Read the model definition and answer for the solid it produces. Units are mm, in the model's axes. A direction names the side the tool comes from. Give positions to 0.01 mm unless a question says otherwise; leave off trailing zeros. Loops run counter-clockwise (first coordinate to the right, second up) from the corner with the lowest first, then second, coordinate; pieces in that order, holes last. Notation, with made-up numbers: M 78,71.25 L 94,71.25 A29 ccw 94,109.25 Z; hole C -30,-38.5 d1. An arc over 180 degrees is marked long. Return JSON: item names as keys, results as strings. Group by question number.
```python
from build123d import *
from build123d.topology import SkipClean

# Parameters (mm, degrees)
BOSS_EXTRUDE1_DEPTH     = 15.875
CUT_EXTRUDE2_START      = -11.875
CUT_EXTRUDE2_DEPTH      = 11.875
M4_CLEARANCE_HOLE1_D    = 4.5
CHAMFER1_SIZE           = 4.7625
SHELL1_OUTLINE_R        = 20.45
SHELL1_DEPTH            = 10.284072775
SHELL1_2_DEPTH          = 2
BOSS_EXTRUDE2_START     = 2
BOSS_EXTRUDE2_DEPTH     = 2
SKETCH7_W               = 7.14375
SKETCH7_H               = 4.7625
SKETCH7_W_2             = 4.7625
SKETCH7_H_2             = 7.14375
CUT_EXTRUDE5_DEPTH      = 0.5
CUT_EXTRUDE7_DEPTH      = 42.774640932
CUT_EXTRUDE7_DEPTH_BACK = 42.774640932
SKETCH9_W               = 6.175
SKETCH9_H               = 19.378
SKETCH9_W_2             = 3.175
SKETCH9_H_2             = 16.378
SKETCH9_W_3             = 1.5018
SKETCH12_R              = 1.27
CUT_EXTRUDE10_DEPTH     = 42.774640932


with BuildPart() as part:
    # Sketch1 → Boss-Extrude1 (new body)
    with BuildSketch(Plane.XY):
        with BuildLine():
            ThreePointArc((-9.919608253, 20.139609532), (-22.45, 0), (-9.919608253, -20.139609532))
            ThreePointArc((-9.919608253, -20.139609532), (-6.265793461, -23.208178662), (-4.449768206, -27.62049453))
            ThreePointArc((-4.449768206, -27.62049453), (0, -31.45), (4.449768206, -27.62049453))
            ThreePointArc((4.449768206, -27.62049453), (6.265793461, -23.208178662), (9.919608253, -20.139609532))
            ThreePointArc((9.919608253, -20.139609532), (22.45, 0), (9.919608253, 20.139609532))
            ThreePointArc((9.919608253, 20.139609532), (6.265793461, 23.208178662), (4.449768206, 27.62049453))
            ThreePointArc((4.449768206, 27.62049453), (0, 31.45), (-4.449768206, 27.62049453))
            ThreePointArc((-4.449768206, 27.62049453), (-6.265793461, 23.208178662), (-9.919608253, 20.139609532))
        make_face()
    extrude(amount=BOSS_EXTRUDE1_DEPTH)

    # Sketch3 → Cut-Extrude2 (cut)
    with SkipClean():  # the faces are left unmerged after this step: merging them gives an invalid solid
        with BuildSketch(Plane.XY.offset(15.875).offset(CUT_EXTRUDE2_START)):
            with BuildLine():
                ThreePointArc((-4.449768206, 27.62049453), (-6.265793461, 23.208178662), (-9.919608253, 20.139609532))
                ThreePointArc((-9.919608253, 20.139609532), (0, 22.45), (9.919608253, 20.139609532))
                ThreePointArc((9.919608253, 20.139609532), (6.265793461, 23.208178662), (4.449768206, 27.62049453))
                ThreePointArc((4.449768206, 27.62049453), (0, 31.45), (-4.449768206, 27.62049453))
            make_face()
            with BuildLine():
                ThreePointArc((9.919608253, -20.139609532), (0, -22.45), (-9.919608253, -20.139609532))
                ThreePointArc((-9.919608253, -20.139609532), (-6.265793461, -23.208178662), (-4.449768206, -27.62049453))
                ThreePointArc((-4.449768206, -27.62049453), (0, -31.45), (4.449768206, -27.62049453))
                ThreePointArc((4.449768206, -27.62049453), (6.265793461, -23.208178662), (9.919608253, -20.139609532))
            make_face()
        extrude(amount=CUT_EXTRUDE2_DEPTH, mode=Mode.SUBTRACT)

    # M4 Clearance Hole1 (through all)
    with Locations(Plane.XY.offset(4)):
        with Locations((0, -26.95), (0, 26.95)):
            Hole(M4_CLEARANCE_HOLE1_D / 2)

    # Chamfer1
    chamfer1_edges = [part.edges().sort_by_distance(p)[0] for p in [
        (22.45, 0, 15.875),
    ]]
    chamfer(chamfer1_edges, length=CHAMFER1_SIZE)

    # Shell1: read off the stored shape, not the designer's step
    # Shell1 outline → Shell1 (cut)
    with SkipClean():  # the faces are left unmerged after this step: merging them gives an invalid solid
        with BuildSketch(Plane.XY):
            Circle(SHELL1_OUTLINE_R)
        extrude(amount=SHELL1_DEPTH, mode=Mode.SUBTRACT)

    # Shell1 2 outline → Shell1 2 (cut)
    with SkipClean():  # the faces are left unmerged after this step: merging them gives an invalid solid
        with BuildSketch(Plane.XY):
            with BuildLine():
                ThreePointArc((-3.336769132, -24.317800965), (0, -22.7), (3.336769132, -24.317800965))
                ThreePointArc((3.336769132, -24.317800965), (5.656595992, -20.826114024), (9.035901505, -18.345434963))
                ThreePointArc((9.035901505, -18.345434963), (0, -20.45), (-9.035901505, -18.345434963))
                ThreePointArc((-9.035901505, -18.345434963), (-5.656595992, -20.826114024), (-3.336769132, -24.317800965))
            make_face()
            with BuildLine():
                ThreePointArc((-3.336769132, 24.317800965), (-5.656595992, 20.826114024), (-9.035901505, 18.345434963))
                ThreePointArc((-9.035901505, 18.345434963), (0, 20.45), (9.035901505, 18.345434963))
                ThreePointArc((9.035901505, 18.345434963), (5.656595992, 20.826114024), (3.336769132, 24.317800965))
                ThreePointArc((3.336769132, 24.317800965), (0, 22.7), (-3.336769132, 24.317800965))
            make_face()
        extrude(amount=SHELL1_2_DEPTH, mode=Mode.SUBTRACT)

    # Shell1 3 outline → Shell1 3 (revolve, cut)
    with SkipClean():  # the faces are left unmerged after this step: merging them gives an invalid solid
        with BuildSketch(Plane.XZ):
            Polygon((16.859072875, 13.875), (0, 13.875), (0, 10.284072775), (20.45, 10.284072775), align=None)
        revolve(axis=Axis((0, 0, 0), (0, 0, 1)), mode=Mode.SUBTRACT)

    # Sketch6 → Boss-Extrude2 (add)
    with SkipClean():  # the faces are left unmerged after this step: merging them gives an invalid solid
        with BuildSketch(Plane(origin=(0, 0, 2), x_dir=(-1, 0, 0), z_dir=(0, 0, -1)).offset(BOSS_EXTRUDE2_START)):
            with BuildLine():
                ThreePointArc((3.336769132, -24.317800965), (0, -22.7), (-3.336769132, -24.317800965))
                ThreePointArc((-3.336769132, -24.317800965), (-5.656595992, -20.826114024), (-9.035901505, -18.345434963))
                ThreePointArc((-9.035901505, -18.345434963), (0, -20.45), (9.035901505, -18.345434963))
                ThreePointArc((9.035901505, -18.345434963), (5.656595992, -20.826114024), (3.336769132, -24.317800965))
            make_face()
            with BuildLine():
                ThreePointArc((-9.035901505, 18.345434963), (-5.656595992, 20.826114024), (-3.336769132, 24.317800965))
                ThreePointArc((-3.336769132, 24.317800965), (0, 22.7), (3.336769132, 24.317800965))
                ThreePointArc((3.336769132, 24.317800965), (5.656595992, 20.826114024), (9.035901505, 18.345434963))
                ThreePointArc((9.035901505, 18.345434963), (0, 20.45), (-9.035901505, 18.345434963))
            make_face()
        extrude(amount=-BOSS_EXTRUDE2_DEPTH)

    # Sketch7 → Cut-Extrude5 (cut)
    with SkipClean():  # the faces are left unmerged after this step: merging them gives an invalid solid
        with BuildSketch(Plane.XY.offset(15.875)):
            with Locations((-5.953125, 0)):
                Rectangle(SKETCH7_W, SKETCH7_H)
            Rectangle(SKETCH7_W_2, SKETCH7_H)
            with Locations((5.953125, 0)):
                Rectangle(SKETCH7_W, SKETCH7_H)
            with Locations((0, -5.953125)):
                Rectangle(SKETCH7_W_2, SKETCH7_H_2)
            with Locations((0, 5.953125)):
                Rectangle(SKETCH7_W_2, SKETCH7_H_2)
        extrude(amount=-CUT_EXTRUDE5_DEPTH, mode=Mode.SUBTRACT)

    # Sketch9 → Cut-Extrude7 (cut, two sides: drawn at the far end of the back side and taken through both)
    # profile 1 of 3: a face of its own
    with SkipClean():  # the faces are left unmerged after this step: merging them gives an invalid solid
        with BuildSketch(Plane(origin=(0, 0, 0), x_dir=(0, 0, -1), z_dir=(1, 0, 0)).offset(-CUT_EXTRUDE7_DEPTH_BACK)):
            with Locations((-4.5893, 0)):
                Rectangle(SKETCH9_W, SKETCH9_H)
            with Locations((-4.5893, 0)):
                Rectangle(SKETCH9_W_2, SKETCH9_H_2, mode=Mode.SUBTRACT)
        # profile 2 of 3: a face of its own
        with BuildSketch(Plane(origin=(0, 0, 0), x_dir=(0, 0, -1), z_dir=(1, 0, 0)).offset(-CUT_EXTRUDE7_DEPTH_BACK)):
            with Locations((-0.7509, 0)):
                Rectangle(SKETCH9_W_3, SKETCH9_H)
        # profile 3 of 3: a face of its own
        with BuildSketch(Plane(origin=(0, 0, 0), x_dir=(0, 0, -1), z_dir=(1, 0, 0)).offset(-CUT_EXTRUDE7_DEPTH_BACK)):
            with Locations((-4.5893, 0)):
                Rectangle(SKETCH9_W_2, SKETCH9_H_2)
        extrude(amount=CUT_EXTRUDE7_DEPTH + CUT_EXTRUDE7_DEPTH_BACK, mode=Mode.SUBTRACT)

    # Sketch12 → Cut-Extrude10 (cut, through all)
    with SkipClean():  # the faces are left unmerged after this step: merging them gives an invalid solid
        with BuildSketch(Plane.XY.offset(15.875)):
            with Locations((-2.55, 11.95)):
                Circle(SKETCH12_R)
            with Locations((2.55, 11.95)):
                Circle(SKETCH12_R)
        extrude(amount=-CUT_EXTRUDE10_DEPTH, mode=Mode.SUBTRACT)


solid = part.part
```
1. Find section C-C (z = 8.75). Write down the section's boundary in (x, y).
2. Find section D-D (y = 11.95). State how many separate pieces and enclosed holes the cut face has, and give its area (3 significant figures).
3. Find section B-B (y = -26.95). Write down the section's boundary in (x, z), and give its area (3 significant figures).
4. The mould has two halves that part along X. Classify faces 1 (the flat face through (21, 0, 7.677)), 2 (the cylindrical face through (6.2, -23.3, 2)), 3 (the cylindrical face through (2.38, 13.21, 14.89)), 4 (the cylindrical face through (-2.72, 13.21, 14.89)): +X half, -X half, draft (parallel to the pull), parting line (faces both ways), or undercut.
5. For faces 5 (the cylindrical face through (0.09, 31.45, 1.97)), 6 (the flat face through (0, 0, 13.875)), 7 (the flat face through (-21, 0, 7.677)), determine the directions among +Z, -Z, +X, -X, +Y, -Y from which every point of the face is accessible in a straight line to the end or side of a thin tool.
6. Flat-ended cylindrical pins translate along their axes: P1, Ø2, axis at x = -21, y = -2, coming from the -Z side; P2, Ø4, axis at x = 7.5, y = -0.5, coming from the +Z side (3 decimals); P3, Ø4, axis at x = -6.5, z = 11, coming from the -Y side; P4, Ø5, axis at x = 1.5, z = 12.5, coming from the -Y side. Find the tip coordinate at first contact, or state that the pin passes through.
7. Find section A-A (z = 3). Write down the section's boundary in (x, y), and give its area (3 significant figures).
8. Straight lines are drawn through the part: line 1 along Y through (x, z) = (0, 1.25); line 2 along Y through (x, z) = (0.5, 7); line 3 along X through (y, z) = (10.5, 2.5). For each, find the intervals that lie inside material, in ascending order.
Result:
{
 "1": {"outline": "C 0,0 d44.9; hole C 0,0 d40.9"},
 "2": {"separate pieces": "3", "enclosed holes": "0", "area": "121 mm2"},
 "3": {"outline": "M -4.57,0 L -2.25,0 L -2.25,4 L -4.57,4 Z; M 2.25,0 L 4.57,0 L 4.57,4 L 2.25,4 Z", "area": "18.6 mm2"},
 "4": {"face 1": "draft", "face 2": "+X half", "face 3": "undercut", "face 4": "undercut"},
 "5": {"face 5": "+Z, -Z, +Y", "face 6": "-Z", "face 7": "-Z, +X, -X"},
 "6": {"P1": "stops at z = 7.68", "P2": "stops at z = 15.875", "P3": "stops at y = -21.99", "P4": "stops at y = -22.45"},
 "7": {"outline": "M -20.25,-9.69 A22.45 ccw -9.92,-20.14 A10 cw -4.45,-27.62 A4.5 ccw 4.45,-27.62 A10 cw 9.92,-20.14 A22.45 ccw 20.25,-9.69 L 18.01,-9.69 A20.45 cw -18.01,-9.69 Z; M -20.25,9.69 L -18.01,9.69 A20.45 cw 18.01,9.69 L 20.25,9.69 A22.45 ccw 9.92,20.14 A10 cw 4.45,27.62 A4.5 ccw -4.45,27.62 A10 cw -9.92,20.14 A22.45 ccw Z; hole C 0,-26.95 d4.5; hole C 0,26.95 d4.5", "area": "334 mm2"},
 "8": {"line 1": "y = -31.45 to -29.2, -24.7 to -20.45, 20.45 to 24.7, 29.2 to 31.45", "line 2": "y = -22.44 to -20.44, 20.44 to 22.44", "line 3": "x = -19.84 to -17.55, 17.55 to 19.84"}
}
